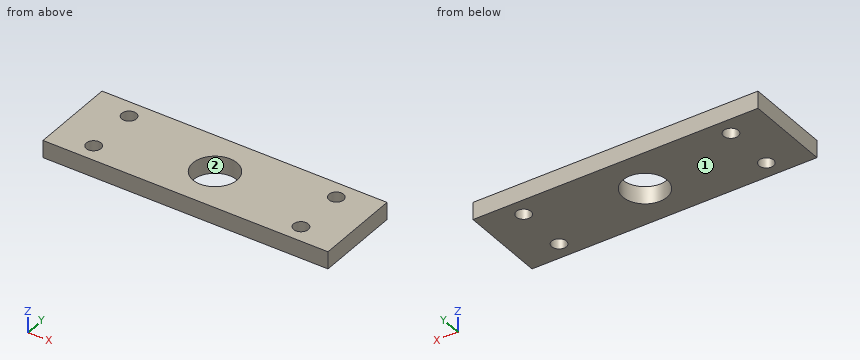
Autodesk Inventor part; units mm, degrees
ref_plane "YZ Plane" through (0, 0, 0) normal (1, 0, 0) x (0, 1, 0)
ref_plane "XZ Plane" through (0, 0, 0) normal (0, 1, 0) x (-1, 0, 0)
ref_plane "XY Plane" through (0, 0, 0) normal (0, 0, 1) x (1, 0, 0)
sketch "Sketch1" plane through (0, 0, 0) normal (0, 0, 1) x (1, 0, 0)
  line L0 (-82.5, 25) -> (82.5, 25)
  line L1 (82.5, 25) -> (82.5, -25)
  line L2 (82.5, -25) -> (-82.5, -25)
  line L3 (-82.5, -25) -> (-82.5, 25)
  circle A0 centre (0, 0) radius 12.8
  circle A1 centre (-60, 15) radius 4.25
  circle A2 centre (-60, -15) radius 4.25
  circle A3 centre (60, 15) radius 4.25
  circle A4 centre (60, -15) radius 4.25
  dimension "d0" = 165
  dimension "d1" = 82.5
  dimension "d2" = 25.6
  dimension "d3" = 50
  dimension "d4" = 25
  dimension "d5" = 8.5
  dimension "d6" = 22.5
  dimension "d7" = 22.5
  dimension "d8" = 22.5
  dimension "d9" = 22.5
  dimension "d10" = 10
  dimension "d11" = 10
  dimension "d12" = 10
  dimension "d13" = 10
extrude "Extrusion1" add sketch "Sketch1" along normal blind 10
properties part number "1222_Former Shaft Plate_V1" material "Aluminum 6061"
Could you check a few things on this model? Use its own coordinates, in mm. Face numbers are marked on the shaded views. Coordinates: 2 decimals unless noted, no trailing zeros. Write each loop counter-clockwise with the first axis right and the second up, starting at its lowest first coordinate (ties: lowest second). Pieces come first, ordered by that corner, then holes. Notation, with made-up numbers: (51, 76.25) - (63, 76.25) arc R17 cw to (63, 100.25) - close; hole circle Ø6 at (-26, 39). An arc over 180 degrees is marked (long way). Write item = value, one per line.
1) We'd pull the mould along Y, two halves only. Please class the marked faces 1 and 2: +Y half, -Y half, draft (parallel to the pull), parting line (faces both ways), or undercut.
Result set:
face_1 = draft
face_2 = undercut
2) Suppose I cut it at D-D on z = 1.5. Please give me the cut outline in (x, y), plus the area to 3 significant figures.
Result set:
outline = (-82.5, -25) - (82.5, -25) - (82.5, 25) - (-82.5, 25) - close; hole circle Ø8.5 at (-60, -15); hole circle Ø8.5 at (-60, 15); hole circle Ø25.6 at (0, 0); hole circle Ø8.5 at (60, -15); hole circle Ø8.5 at (60, 15)
area = 7,510 mm2
3) Suppose I cut it at B-B on y = 0. Please give me the cut outline in (x, z).
Result set:
outline = (-82.5, 0) - (-12.8, 0) - (-12.8, 10) - (-82.5, 10) - close; (12.8, 0) - (82.5, 0) - (82.5, 10) - (12.8, 10) - close
4) Suppose I cut it at A-A on y = 15. Please give me the cut outline in (x, z), plus the area to 3 significant figures.
Result set:
outline = (-82.5, 0) - (-64.25, 0) - (-64.25, 10) - (-82.5, 10) - close; (-55.75, 0) - (55.75, 0) - (55.75, 10) - (-55.75, 10) - close; (64.25, 0) - (82.5, 0) - (82.5, 10) - (64.25, 10) - close
area = 1,480 mm2
5) Will this pin go through, and if not, where does the flat tip stop? pin 1 Ø5 at (x, y) = (-31.5, -15) entering from -Z.
Result set:
pin_1 = 0
6) Suppose I cut it at C-C on x = 60. Please give me the cut outline in (y, z).
Result set:
outline = (-25, 0) - (-19.25, 0) - (-19.25, 10) - (-25, 10) - close; (-10.75, 0) - (10.75, 0) - (10.75, 10) - (-10.75, 10) - close; (19.25, 0) - (25, 0) - (25, 10) - (19.25, 10) - close
7) Please list where these lines run through material, in increasing order: line 1 (Y direction, x = -60, z = 3.25); line 2 (X direction, y = 14, z = 5.5); line 3 (X direction, y = -17.5, z = 1.25). Write a range as [from, to].
Result set:
line_1 = [-25, -19.25], [-10.75, 10.75], [19.25, 25]
line_2 = [-82.5, -64.13], [-55.87, 55.87], [64.13, 82.5]
line_3 = [-82.5, -63.44], [-56.56, 56.56], [63.44, 82.5]
